Here's the drawing with two shaded views (mm, measured from the low corner). I have some questions. Round coordinates to 2 decimals unless told otherwise and drop trailing zeros. Write each loop counter-clockwise with the first axis right and the second up, starting at its lowest first coordinate (ties: lowest second). Pieces come first, ordered by that corner, then holes. Notation, with made-up numbers: M 8,-20.5 L 14,-20.5 A29 ccw 14,14.5 Z; hole C 23,42.25 d4. An arc over 180 degrees is marked long. Answer as a JSON object with one key per item and string values. Group by question number.
1) Suppose I cut it at C-C, the plane x = 24.5. Write out the boundary of the cut face in (y, z).
2) If we mould it in two halves opening along X, with no side actions, what happens to the marked faces 1, 2 and 3? For each: +X half, -X half, draft (parallel to the pull), parting line (faces both ways), or undercut.
3) I'm going to push flat-ended pins straight in: pin 1 Ø15 at (x, z) = (221, 2170.5) entering from -Y; pin 2 Ø3 at (x, z) = (199.5, 1965.5) entering from -Y; pin 3 Ø4 at (x, z) = (94, 2136) entering from +Y; pin 4 Ø19 at (y, z) = (42.5, 2135) entering from +X. Where does each tip first touch, or does it pass through?
4) Please list where these lines run through material, in increasing order: L1, parallel to Z at x = 153.5, y = 55.5; L2, parallel to X at y = 65, z = 1733; L3, parallel to Y at x = 71, z = 996. Write a range as [from, to].
5) Suppose I cut it at B-B, the plane z = 2120. Write out the boundary of the cut face in (x, y), and give its area (3 significant figures).
6) Suppose I cut it at D-D, the plane z = 499.5. Write out the boundary of the cut face in (x, y).
7) Suppose I cut it at A-A, the plane x = 149.5. Write out the boundary of the cut face in (y, z).
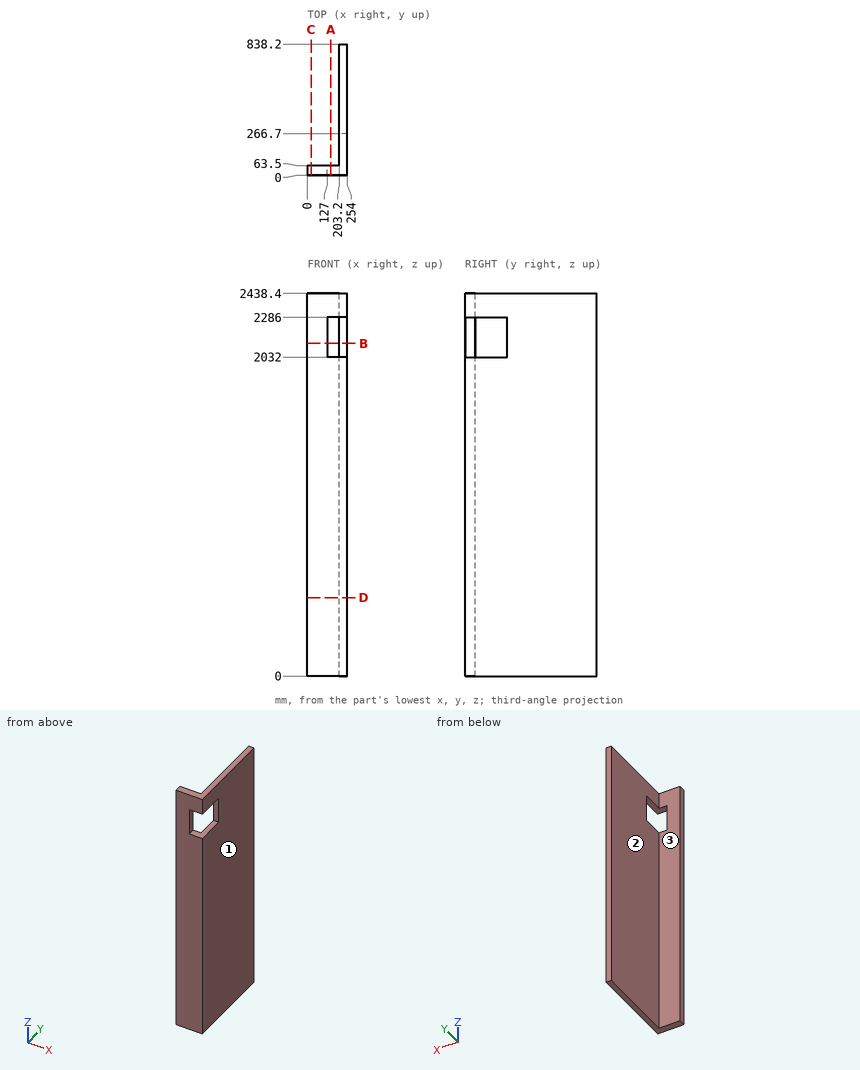
Results:
{
 "1": {"outline": "M 0,0 L 63.5,0 L 63.5,2438.4 L 0,2438.4 Z"},
 "2": {"face 1": "+X half", "face 2": "-X half", "face 3": "draft"},
 "3": {"pin 1": "y = 266.7", "pin 2": "y = 0", "pin 3": "y = 63.5", "pin 4": "x = 127"},
 "4": {"L1": "[0, 2032], [2286, 2438.4]", "L2": "[203.2, 254]", "L3": "[0, 63.5]"},
 "5": {"outline": "M 0,0 L 127,0 L 127,63.5 L 0,63.5 Z; M 203.2,266.7 L 254,266.7 L 254,838.2 L 203.2,838.2 Z", "area": "37,100 mm^2"},
 "6": {"outline": "M 0,0 L 254,0 L 254,838.2 L 203.2,838.2 L 203.2,63.5 L 0,63.5 Z"},
 "7": {"outline": "M 0,0 L 63.5,0 L 63.5,2032 L 0,2032 Z; M 0,2286 L 63.5,2286 L 63.5,2438.4 L 0,2438.4 Z"}
}
